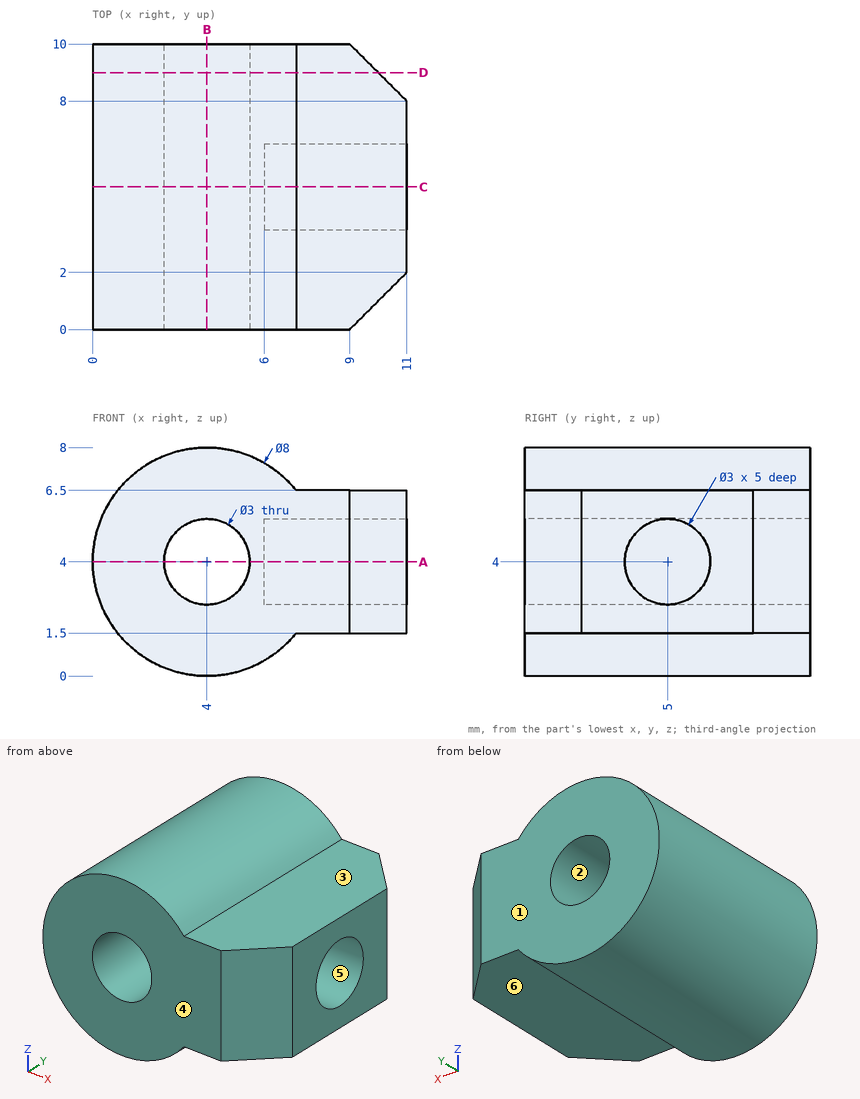
Geometry check sheet. Reference: drawing and pictorial views, mm from the part's lowest x, y, z. A direction names the side the tool comes from. Give positions to 0.01 mm unless a question says otherwise; leave off trailing zeros. Order: outer loops, then holes, each group sorted by start corner. A loop starts at its lowest first (then second) coordinate and runs counter-clockwise, first axis right, second up. Notation, with made-up numbers: (53.25, 58) -> (91.25, 58) arc R29 ccw to (91.25, 89) -> close; hole circle Ø4 at (-34, 2). An arc over 180 degrees is marked (long way). Write each question's results on one line, items separated by ' | '. Start each with the question number.
(1) Sectioned sample at D-D (y = 9). Enter the section's corners in (x, z), plus the area to 3 significant figures.
(2) Sectioned sample at A-A (z = 4). Enter the section's corners in (x, y), plus the area to 3 significant figures.
(3) Access from +Z, -Z, +X, -X, +Y, -Y to the whole of each face (thin tool, end or side, straight path). Record for the marked faces 4, 5 and 6.
(4) Sectioned sample at C-C (y = 5). Enter the section's corners in (x, z).
(5) Mould release check, pull along Z, two halves, no side actions. Record for the marked faces 1, 2 and 3: pulls with the +Z half, pulls with the -Z half, needs draft (parallel to the pull), parting line crosses it, or undercut.
(6) Sectioned sample at B-B (x = 4). Enter the section's corners in (y, z), plus the area to 3 significant figures.
(7) Gauge pin test, flat ends, axial feed: P1, Ø2, axis at x = 7.5, y = 3, coming from the +Z side; P2, Ø3, axis at y = 4.5, z = 7, coming from the -X side; P3, Ø4.5, axis at x = 8.5, y = 4.5, coming from the +Z side. Record the tip position at first contact, or that the pin passes through.
(8) Scan lines: line 1 (X direction, y = 6, z = 4); line 2 (Z direction, x = 8.2, y = 5); line 3 (X direction, y = 6.75, z = 4). Record each from-to range of solid material in increasing order.
Answer below:
1) outline: (7.12, 1.5) -> (10, 1.5) -> (10, 6.5) -> (7.12, 6.5) arc R4 ccw (long way) to start; hole circle Ø3 at (4, 4) | area: 54.6 mm2
2) outline: (0, 0) -> (2.5, 0) -> (2.5, 10) -> (0, 10) -> close; (5.5, 0) -> (9, 0) -> (11, 2) -> (11, 3.5) -> (6, 3.5) -> (6, 6.5) -> (11, 6.5) -> (11, 8) -> (9, 10) -> (5.5, 10) -> close | area: 61.0 mm2
3) face 4: +Z, -Z, +X, -X, -Y | face 5: +X | face 6: -Z, +X, +Y, -Y
4) outline: (6, 2.5) -> (6, 5.5) -> (11, 5.5) -> (11, 6.5) -> (7.12, 6.5) arc R4 ccw (long way) to (7.12, 1.5) -> (11, 1.5) -> (11, 2.5) -> close; hole circle Ø3 at (4, 4)
5) face 1: needs draft | face 2: undercut | face 3: pulls with the +Z half
6) outline: (0, 0) -> (10, 0) -> (10, 2.5) -> (0, 2.5) -> close; (0, 5.5) -> (10, 5.5) -> (10, 8) -> (0, 8) -> close | area: 50.0 mm2
7) P1: z = 7.12 | P2: x = 0.29 | P3: z = 7.31
8) line 1: 0 to 2.5, 5.5 to 6 | line 2: 1.5 to 2.5, 5.5 to 6.5 | line 3: 0 to 2.5, 5.5 to 11
